For this review, take the finished solid that the model builds, in its own axes (mm). Coordinates: 2 decimals unless noted, no trailing zeros. Write each loop counter-clockwise with the first axis right and the second up, starting at its lowest first coordinate (ties: lowest second). Pieces come first, ordered by that corner, then holes. Notation, with made-up numbers: M 89.5,-16 L 142.5,-16 A19 ccw 142.5,15 Z; hole C -20.75,56.25 d1. An arc over 180 degrees is marked long. One line per question, with ' | ' between items.
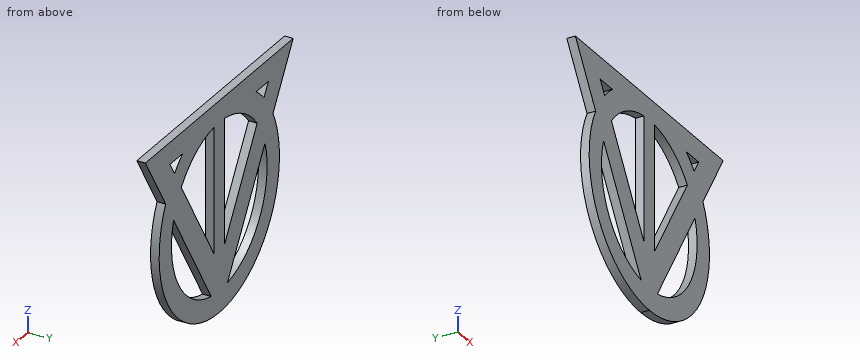
from build123d import *

# Parameters (mm, degrees)
F1_DEPTH = 2.54


with BuildPart() as f1:
    # F0 (on Front) → F1 (new body)
    with BuildSketch(Plane.XZ):
        with BuildLine():
            Line((-28.245696, 21.590037), (-17.819697, 4.609524))
            ThreePointArc((-17.819697, 4.609524), (-16.568917, -25.598129), (9.804215, -40.380711))
            ThreePointArc((9.804215, -40.380711), (9.829259, -40.380741), (9.854304, -40.380751))
            ThreePointArc((9.854304, -40.380751), (9.879348, -40.380741), (9.904392, -40.380711))
            ThreePointArc((9.904392, -40.380711), (36.277524, -25.598129), (37.528304, 4.609524))
            Line((37.528304, 4.609524), (47.954304, 21.590037))
            Line((47.954304, 21.590037), (11.468784, 21.590037))
            Line((11.468784, 21.590037), (9.854304, 21.590037))
            Line((9.854304, 21.590037), (8.239823, 21.590037))
            Line((8.239823, 21.590037), (-28.245696, 21.590037))
        make_face()
        with BuildLine():
            ThreePointArc((5.687621, -33.676138), (-11.15754, -22.275555), (-13.703103, -2.095048))
            Line((-13.703103, -2.095048), (5.687621, -33.676138))
        make_face(mode=Mode.SUBTRACT)
        with BuildLine():
            ThreePointArc((33.41171, -2.095048), (30.866148, -22.275555), (14.020986, -33.676138))
            Line((14.020986, -33.676138), (33.41171, -2.095048))
        make_face(mode=Mode.SUBTRACT)
        with BuildLine():
            Line((7.10099, -21.646665), (-9.674308, 5.678003))
            ThreePointArc((-9.674308, 5.678003), (-2.247189, 12.108065), (7.10099, 15.127888))
            Line((7.10099, 15.127888), (7.10099, -21.646665))
        make_face(mode=Mode.SUBTRACT)
        with BuildLine():
            Line((-13.177649, 11.384468), (-15.480497, 15.135492))
            Line((-15.480497, 15.135492), (-9.136935, 15.135492))
            ThreePointArc((-9.136935, 15.135492), (-11.240831, 13.34997), (-13.177649, 11.384468))
        make_face(mode=Mode.SUBTRACT)
        with BuildLine():
            ThreePointArc((12.550589, 15.13423), (21.982633, 12.092926), (29.455338, 5.583573))
            Line((29.455338, 5.583573), (12.550589, -21.951937))
            Line((12.550589, -21.951937), (12.550589, 15.13423))
        make_face(mode=Mode.SUBTRACT)
        with BuildLine():
            Line((28.845543, 15.135492), (35.319503, 15.135492))
            Line((35.319503, 15.135492), (32.963703, 11.298217))
            ThreePointArc((32.963703, 11.298217), (30.991879, 13.310498), (28.845543, 15.135492))
        make_face(mode=Mode.SUBTRACT)
    extrude(amount=F1_DEPTH)


solid = f1.part
1) We need section D-D on z = -9. State the section outline as (x, y) points, then the cut area to 3 significant figures.
Responses:
outline: M -21.15,-2.54 L -14.8,-2.54 L -14.8,0 L -21.15,0 Z; M -9.46,-2.54 L -0.66,-2.54 L -0.66,0 L -9.46,0 Z; M 7.1,-2.54 L 12.55,-2.54 L 12.55,0 L 7.1,0 Z; M 20.5,-2.54 L 29.17,-2.54 L 29.17,0 L 20.5,0 Z; M 34.51,-2.54 L 40.86,-2.54 L 40.86,0 L 34.51,0 Z | area: 90.5 mm^2
2) Insertion check: pin 1 Ø0.8 at (y, z) = (-1, 4) entering from -X; pin 2 Ø1.3 at (x, y) = (-12.5, -1) entering from -Z. Each pin has a flat end and moves straight along its axis. Give the tip position at first contact, or say it passes through.
Responses:
pin 1: x = -18.31 | pin 2: z = -31.52
3) We need section B-B on x = 32. State the section outline as (y, z) points, then the cut area to 3 significant figures.
Responses:
outline: M -2.54,-31.08 L 0,-31.08 L 0,-20.21 L -2.54,-20.21 Z; M -2.54,-4.39 L 0,-4.39 L 0,12.33 L -2.54,12.33 Z; M -2.54,15.14 L 0,15.14 L 0,21.59 L -2.54,21.59 Z | area: 86.5 mm^2
4) To check wall thickness, follow line 1 along Z through (x, y) = (0, -1.85); line 2 along X through (y, z) = (-0.8, -19); line 3 along Z through (x, y) = (-8, -2). State the ranges of each line that lie inside material, in increasing order. Write a range as [from, to].
Responses:
line 1: [-38.77, -31.98], [-24.41, -10.08], [13.23, 21.59] | line 2: [-19.62, -12.85], [-3.32, 5.48], [7.1, 12.55], [14.36, 23.03], [32.55, 39.33] | line 3: [-34.72, -26.38], [-11.38, 2.95], [7.63, 21.59]
5) We need section A-A on y = -0.75. State the section outline as (x, z) points.
Responses:
outline: M -28.25,21.59 L -17.82,4.61 A31.01 ccw 9.8,-40.38 A31.36 ccw 9.9,-40.38 A31.01 ccw 37.53,4.61 L 47.95,21.59 Z; hole M -15.48,15.14 L -13.18,11.38 A31.01 cw -9.14,15.14 Z; hole M -13.7,-2.1 A24.66 ccw 5.69,-33.68 Z; hole M -9.67,5.68 L 7.1,-21.65 L 7.1,15.13 A24.66 ccw Z; hole M 12.55,-21.95 L 29.46,5.58 A24.66 ccw 12.55,15.13 Z; hole M 14.02,-33.68 A24.66 ccw 33.41,-2.1 Z; hole M 28.85,15.14 A31.01 cw 32.96,11.3 L 35.32,15.14 Z
6) We need section C-C on z = 0.5. State the section outline as (x, y) points.
Responses:
outline: M -19.54,-2.54 L -6.5,-2.54 L -6.5,0 L -19.54,0 Z; M 7.1,-2.54 L 12.55,-2.54 L 12.55,0 L 7.1,0 Z; M 26.33,-2.54 L 39.25,-2.54 L 39.25,0 L 26.33,0 Z
